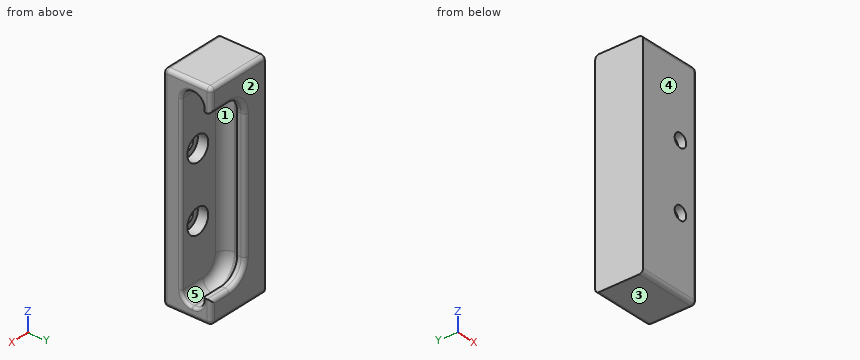
Autodesk Inventor part; units mm, degrees
ref_plane "YZ Plane" through (0, 0, 0) normal (1, 0, 0) x (0, 1, 0)
ref_plane "XZ Plane" through (0, 0, 0) normal (0, 1, 0) x (-1, 0, 0)
ref_plane "XY Plane" through (0, 0, 0) normal (0, 0, 1) x (1, 0, 0)
sketch "Sketch1" plane through (0, 0, 0) normal (0, 1, 0) x (-1, 0, 0)
  circle A0 centre (0, 12.5) radius 2.6
  circle A1 centre (0, -12.5) radius 2.6
  circle A2 centre (0, 12.5) radius 4.75
  circle A3 centre (0, -12.5) radius 4.75
  circle A4 centre (0, 12.5) radius 7.5
  circle A5 centre (0, -12.5) radius 7.5
  line L0 (7.5, 12.5) -> (7.5, -12.5)
  line L1 (-7.5, -12.5) -> (-7.5, 12.5)
  line L2 (0, 12.5) -> (0, -12.5) construction
  line L3 (7.5, -12.5) -> (7.5, 12.5)
  line L4 (-7.5, 41) -> (17, 41)
  line L5 (17, 41) -> (17, -41)
  line L6 (17, -41) -> (-7.5, -41)
  line L7 (-7.5, -41) -> (-7.5, 41)
  point P0 (0, 0)
  point P1 (7.5, -41)
  dimension "d0" = 5.2
  dimension "d1" = 5.2
  dimension "d2" = 25
  dimension "d3" = 12.5
  dimension "d6" = 9.5
  dimension "d7" = 9.5
  dimension "d8" = 15
  dimension "d9" = 15
  dimension "d19" = 24.5
  dimension "d20" = 82
  dimension "d21" = 41
extrude "Extrusion1" add sketch "Sketch1" along normal blind 3 contours A2 | A3
extrude "Extrusion2" add sketch "Sketch1" along normal blind 7 contours A4 | L0 A5 L1 A4 | A4 L7 L4 L5 L6 A5 L0 | A5
sketch "Sketch2" plane through (0, 7, 0) normal (0, 1, 0) x (1, 0, 0)
  circle A0 centre (0, 12.5) radius 4.75
  circle A1 centre (0, -12.5) radius 4.75
  line L0 (-17, -41) -> (7.5, -41)
  line L1 (7.5, -41) -> (7.5, 41)
  line L2 (7.5, 41) -> (-17, 41)
  line L3 (-17, 41) -> (-17, -41)
  line L4 (7.5, 41) -> (7.5, -41)
  line L5 (7.5, -37) -> (-2.3, -37)
  line L6 (-12, -27.3) -> (-12, 27.3)
  line L7 (7.5, 37) -> (-2.3, 37)
  arc A2 (-12, -27.3) -> (-2.3, -37) centre (-2.3, -27.3) ccw
  arc A3 (-2.3, 37) -> (-12, 27.3) centre (-2.3, 27.3) ccw
  point P0 (0, 0)
  dimension "d23" = 5
  dimension "d24" = 4
  dimension "d25" = 4
  dimension "d26" = 9.7
extrude "Extrusion3" add sketch "Sketch2" along normal blind 8.4 contours L3 L2 L1 L7 A3 L6 A2 L5 L0
sketch "Sketch3" plane through (0, 15.4, 0) normal (0, 1, 0) x (1, 0, 0)
  line L0 (7.5, -41) -> (7.5, -37)
  line L1 (7.5, -37) -> (-2.3, -37)
  arc A0 (-12, -27.3) -> (-2.3, -37) centre (-2.3, -27.3) ccw
  line L2 (-12, -27.3) -> (-12, 27.3)
  arc A1 (-2.3, 37) -> (-12, 27.3) centre (-2.3, 27.3) ccw
  line L3 (-2.3, 37) -> (7.5, 37)
  line L4 (7.5, 37) -> (7.5, 41)
  line L5 (7.5, 41) -> (-17, 41)
  line L6 (-17, 41) -> (-17, -41)
  line L7 (-17, -41) -> (7.5, -41)
  line L8 (7.5, -37) -> (7.5, 37)
  line L9 (7.5, -32) -> (-0.75, -32)
  line L10 (7.5, 32) -> (-0.75, 32)
  line L11 (-8, -24.75) -> (-8, 24.75)
  arc A2 (-8, -24.75) -> (-0.75, -32) centre (-0.75, -24.75) ccw
  arc A3 (-0.75, 32) -> (-8, 24.75) centre (-0.75, 24.75) ccw
  line L12 (7.5, -32) -> (7.5, -37)
  line L13 (7.5, 32) -> (7.5, 37)
  point P0 (0, 0)
  dimension "d29" = 64
  dimension "d30" = 32
  dimension "d31" = 4
  dimension "d32" = 7.25
extrude "Extrusion4" add sketch "Sketch3" along normal blind 3 contours L7 L6 L5 L4 L3 A1 L2 A0 L1 L0 | L1 A0 L2 A1 L3 L8 L10 A3 L11 A2 L9
fillet "Fillet1" radius 4 5 edges at (2.6, 7, 37) (-12, 7, 0) (-9.1589, 7, -34.1589) (2.6, 7, -37) (-9.1589, 7, 34.1589)
fillet "Fillet2" radius 4 5 edges at (-12, 15.4, 0) (-9.1589, 15.4, -34.1589) (2.6, 15.4, -37) (2.6, 15.4, 37) (-9.1589, 15.4, 34.1589)
fillet "Fillet3" radius 1 3 edges at (7.5, 7, 0) (7.5, 8.1716, -35.8284) (7.5, 8.1716, 35.8284)
fillet "Fillet4" radius 1.5 14 edges at (-5.8765, 18.4, 29.8765) (-8, 18.4, 0) (-5.8765, 18.4, -29.8765) (3.375, 18.4, -32) (3.375, 18.4, 32) (7.5, 18.4, 36.5) (-4.75, 18.4, -41) (-4.75, 18.4, 41) (7.5, 18.4, -36.5) (7.5, 9.2, -41) (7.5, 9.2, 41) (-4.75, 0, 41) (7.5, 0, 0) (-4.75, 0, -41)
properties part number "HolderFront"
Input: part model. Units: mm. Frame: model coordinates. Face numbers are marked on the shaded views. A direction names the side the tool comes from. Coordinates: 2 decimals unless noted, no trailing zeros. Write each loop counter-clockwise with the first axis right and the second up, starting at its lowest first coordinate (ties: lowest second). Pieces come first, ordered by that corner, then holes. Notation, with made-up numbers: (53, -15.75) -> (86, -15.75) arc R11 cw to (86, 2.25) -> close; hole circle Ø8 at (-6, 6.5). An arc over 180 degrees is marked (long way). Answer as a JSON object with one key per item and string values.
1. Section B-B on y = 2.25. Return the cut outline in (x, z), then the cut area to 3 significant figures.
Result set:
{"outline": "(-17, -41) -> (6, -41) arc R1.5 ccw to (7.5, -39.5) -> (7.5, 39.5) arc R1.5 ccw to (6, 41) -> (-17, 41) -> close; hole circle Ø5.2 at (0, -12.5); hole circle Ø5.2 at (0, 12.5)", "area": "1,970 mm2"}
2. First-contact query: P1, Ø8.5, axis at x = 0, z = 12.5, coming from the +Y side; P2, Ø11.5, axis at x = -3, z = 7.5, coming from the -Y side; P3, Ø7, axis at x = 2.5, z = -14, coming from the +Y side; P4, Ø1.2, axis at y = 16.5, z = 11, coming from the +X side. Flat tips, straight axial feed; report the tip coordinate or a pass-through.
Result set:
{"P1": "stops at y = 3", "P2": "stops at y = 0", "P3": "stops at y = 7", "P4": "stops at x = -8"}
3. Material intervals for line 1 (Z direction, x = 0, y = 5.55); line 2 (Z direction, x = 0, y = 2.4); line 3 (Y direction, x = -0.5, z = -17.5), sorted ascending. Write a range as from..to.
Result set:
{"line 1": "z = -41..-17.25, -7.75..7.75, 17.25..41", "line 2": "z = -41..-15.1, -9.9..9.9, 15.1..41", "line 3": "y = 0..7"}
4. Access query for the marked faces 1 and 2. Directions: +Z, -Z, +X, -X, +Y, -Y. A direction counts if a zero-diameter tool reaches every point of the face in a straight line with its end or side. Return the directions, or none.
Result set:
{"face 1": "+X", "face 2": "+Z, -Z, +X, -X, +Y"}
5. Mould query, pull axis Z, two halves, no side actions, for the marked faces 3, 4 and 5. Classes: released by +Z, released by -Z, zero draft, split by the parting line, or undercut.
Result set:
{"face 3": "released by -Z", "face 4": "zero draft", "face 5": "undercut"}
6. Section D-D on x = 0. Count the separate pieces of the cut face and the enclosed holes in it, then the cut area to 3 significant figures.
Result set:
{"separate pieces": "3", "enclosed holes": "0", "area": "599 mm2"}
